Source: CAD feature listing. Evaluate the final solid. Frame: model axes, mm. A direction names the side the tool comes from. Give positions to 0.01 mm unless a question says otherwise; leave off trailing zeros. Order: outer loops, then holes, each group sorted by start corner. A loop starts at its lowest first (then second) coordinate and runs counter-clockwise, first axis right, second up. Notation, with made-up numbers: M -32,68 L 6,68 A10 ccw 6,87 Z; hole C 34.5,-3.75 d7. An arc over 180 degrees is marked long. Return JSON: item names as keys, results as strings.
from build123d import *

# Parameters (mm, degrees)
F0_R     = 1.5875
F1_DEPTH = 1.778
F2_W     = 13.335
F2_H     = 8.89
F3_DEPTH = 9.525
F4_W     = 15.875
F4_H     = 12.7
F5_DEPTH = 9.525


with BuildPart() as f1:
    # F0 (on Front) → F1 (new body)
    with BuildSketch(Plane.XZ):
        Polygon((0, 53.34), (0, 0), (66.58718, 0), (66.58718, 2.54), (70.5304, 5.08), (70.5304, 37.846), (66.735297, 40.386), (66.735297, 51.816), (64.516, 53.34), align=None)
        with Locations((13.97, 2.54)):
            Circle(F0_R, mode=Mode.SUBTRACT)
        with Locations((66.04, 7.62)):
            Circle(F0_R, mode=Mode.SUBTRACT)
        with Locations((15.24, 50.8)):
            Circle(F0_R, mode=Mode.SUBTRACT)
        with Locations((66.04, 35.56)):
            Circle(F0_R, mode=Mode.SUBTRACT)
    extrude(amount=F1_DEPTH)

    # F2 (on face) → F3 (join)
    with BuildSketch(Plane.XZ.offset(1.778)):
        with Locations((4.7625, 7.62)):
            Rectangle(F2_W, F2_H)
    extrude(amount=F3_DEPTH)

    # F4 (on face) → F5 (join)
    with BuildSketch(Plane.XZ.offset(1.778)):
        with Locations((1.5875, 38.735)):
            Rectangle(F4_W, F4_H)
    extrude(amount=F5_DEPTH)


solid = f1.part
1. Section query C-C (x = 6.5). Return loops of the section in (y, z) (3 decimals), then the cut area to 3 significant figures.
Evaluation:
{"outline": "M -11.303,3.175 L -1.778,3.175 L -1.778,0 L 0,0 L 0,53.34 L -1.778,53.34 L -1.778,45.085 L -11.303,45.085 L -11.303,32.385 L -1.778,32.385 L -1.778,12.065 L -11.303,12.065 Z", "area": "300 mm^2"}
2. Section query A-A (z = 7.62). Return loops of the section in (x, y) (1 decimal).
Evaluation:
{"outline": "M -1.9,-11.3 L 11.4,-11.3 L 11.4,-1.8 L 64.5,-1.8 L 64.5,0 L 0,0 L 0,-1.8 L -1.9,-1.8 Z; M 67.6,-1.8 L 70.5,-1.8 L 70.5,0 L 67.6,0 Z"}
3. Set-up query: faces 4 (the face through (1, -6, 32.385)), 5 (the face through (-1.905, -6, 8)), 6 (the face through (0, -1, 27)). Return all of +Z, -Z, +X, -X, +Y, -Y with unobstructed straight access to the full face (end or side cutting, diameter ignored); none if empty.
Evaluation:
{"face 4": "+X, -X, -Y", "face 5": "-Z, -X, +Y, -Y", "face 6": "+Z, -Z, -X, +Y"}
4. Ray query, probe 1 along Z at (x, y) = (15.24, -1.35); probe 2 along Z at (x, y) = (3, -8.25) (3 decimals); probe 3 along Z at (x, y) = (66.04, -1). Return the intervals inside material, ascending.
Evaluation:
{"probe 1": "z = 0 to 1.59, 3.49 to 49.21, 52.39 to 53.34", "probe 2": "z = 3.175 to 12.065, 32.385 to 45.085", "probe 3": "z = 0 to 6.03, 9.21 to 33.97, 37.15 to 52.29"}
5. Section query B-B (y = -10). Return loops of the section in (x, z) (3 decimals).
Evaluation:
{"outline": "M -6.35,32.385 L 9.525,32.385 L 9.525,45.085 L -6.35,45.085 Z; M -1.905,3.175 L 11.43,3.175 L 11.43,12.065 L -1.905,12.065 Z"}
6. First-contact query: pin 1 (3 mm diameter, centred on x = 5.5, y = -5.5, fed in from -Z) (3 decimals); pin 2 (5 mm diameter, centred on x = 59.5, y = -5.5, fed in from +Z); pin 3 (0.9 mm diameter, centred on y = -1.5, z = 46.5, fed in from +X); pin 4 (3 mm diameter, centred on x = 2, y = -5.5, fed in from +Z) (3 decimals). Flat tips, straight axial feed; report the tip coordinate or a pass-through.
Evaluation:
{"pin 1": "stops at z = 3.175", "pin 2": "passes through", "pin 3": "stops at x = 66.74", "pin 4": "stops at z = 45.085"}
7. Section query D-D (z = 50.8). Return loops of the section in (x, y), then the cut area to 3 significant figures.
Evaluation:
{"outline": "M 0,-1.78 L 13.65,-1.78 L 13.65,0 L 0,0 Z; M 16.83,-1.78 L 66.74,-1.78 L 66.74,0 L 16.83,0 Z", "area": "113 mm^2"}
8. Draft query along Z for faces 1 (the face through (5, -6, 12.065)), 2 (the face through (68.53, -0.88, 3.79)), 3 (the face through (9.525, -6, 39)). Return one class per face: pulls with the +Z half, pulls with the -Z half, needs draft (parallel to the pull), parting line crosses it, or undercut.
Evaluation:
{"face 1": "undercut", "face 2": "pulls with the -Z half", "face 3": "needs draft"}
